Geometry: final body of the model. Coordinates: model frame, mm. A direction names the side the tool comes from. Give positions to 0.01 mm unless a question says otherwise; leave off trailing zeros. Loops run counter-clockwise (first coordinate to the right, second up) from the corner with the lowest first, then second, coordinate; pieces in that order, holes last.
1. Material intervals for line 1 along X through (y, z) = (-1260, -5); line 2 along Z through (x, y) = (1, -91.5); line 3 along X through (y, z) = (-276.5, 27), sorted ascending.
2. Section A-A, the plane y = -488. Output: boundary loops of the cut face in (x, z).
3. Draft query along X for faces 1 (the face through (-1, -701, -15.773)), 2 (the face through (-30.121, -701, 7)), 3 (the face through (-1, -701, 35.027)). Return one class per face: +X half, -X half, draft (parallel to the pull), parting line (faces both ways), or undercut.
4. Section C-C, the plane x = -11. Output: boundary loops of the cut face in (y, z), then the cut area to 3 significant figures.
5. Access query for faces 4 (the face through (23, -1422.4, 7)), 5 (the face through (20.679, -701, 8)). Directions: +Z, -Z, +X, -X, +Y, -Y. A direction counts if a zero-diameter tool reaches every point of the face in a straight line with its end or side. Return the directions, or none.
6. Section B-B, the plane z = -0.5. Output: boundary loops of the cut face in (x, y), then the cut area to 3 significant figures.
from build123d import *

# Parameters (mm, degrees)
F1_DEPTH = 1422.4


with BuildPart() as f1:
    # F0 (on Front) → F1 (new body)
    with BuildSketch(Plane.XZ):
        with BuildLine():
            Line((24.488532, 35.02659), (-27.581468, 35.02659))
            ThreePointArc((-27.581468, 35.02659), (-29.377519, 34.282641), (-30.121468, 32.48659))
            Line((-30.121468, 32.48659), (-30.121468, -19.58341))
            ThreePointArc((-30.121468, -19.58341), (-29.377519, -21.379462), (-27.581468, -22.12341))
            Line((-27.581468, -22.12341), (24.488532, -22.12341))
            ThreePointArc((24.488532, -22.12341), (26.284584, -21.379462), (27.028532, -19.58341))
            Line((27.028532, -19.58341), (27.028532, 32.48659))
            ThreePointArc((27.028532, 32.48659), (26.284584, 34.282641), (24.488532, 35.02659))
        make_face()
        with BuildLine():
            ThreePointArc((-23.771468, 26.13659), (-23.027519, 27.932641), (-21.231468, 28.67659))
            Line((-21.231468, 28.67659), (20.678532, 28.67659))
            Line((20.678532, 28.67659), (20.678532, -13.23341))
            ThreePointArc((20.678532, -13.23341), (19.934584, -15.029462), (18.138532, -15.77341))
            Line((18.138532, -15.77341), (-21.231468, -15.77341))
            ThreePointArc((-21.231468, -15.77341), (-23.027519, -15.029462), (-23.771468, -13.23341))
            Line((-23.771468, -13.23341), (-23.771468, 26.13659))
        make_face(mode=Mode.SUBTRACT)
    extrude(amount=F1_DEPTH)


solid = f1.part
Answers below:
1. line 1: x = -30.12 to -23.77, 20.68 to 27.03
1. line 2: z = -22.12 to -15.77, 28.68 to 35.03
1. line 3: x = -30.12 to -23.62, 20.68 to 27.03
2. outline: (-30.12, -19.58) arc R2.54 ccw to (-27.58, -22.12) - (24.49, -22.12) arc R2.54 ccw to (27.03, -19.58) - (27.03, 32.49) arc R2.54 ccw to (24.49, 35.03) - (-27.58, 35.03) arc R2.54 ccw to (-30.12, 32.49) - close; hole (-23.77, -13.23) arc R2.54 ccw to (-21.23, -15.77) - (18.14, -15.77) arc R2.54 ccw to (20.68, -13.23) - (20.68, 28.68) - (-21.23, 28.68) arc R2.54 ccw to (-23.77, 26.14) - close
3. face 1: undercut
3. face 2: -X half
3. face 3: draft
4. outline: (-1422.4, -22.12) - (0, -22.12) - (0, -15.77) - (-1422.4, -15.77) - close; (-1422.4, 28.68) - (0, 28.68) - (0, 35.03) - (-1422.4, 35.03) - close
4. area: 18,100 mm2
5. face 4: +Z, -Z, +X, -X, -Y
5. face 5: +Y, -Y
6. outline: (-30.12, -1422.4) - (-23.77, -1422.4) - (-23.77, 0) - (-30.12, 0) - close; (20.68, -1422.4) - (27.03, -1422.4) - (27.03, 0) - (20.68, 0) - close
6. area: 18,100 mm2
